CAD build for the part. Positions are in the model's coordinates, mm. A direction names the side the tool comes from. Round coordinates to 2 decimals unless told otherwise and drop trailing zeros. Loops run counter-clockwise (first coordinate to the right, second up) from the corner with the lowest first, then second, coordinate; pieces in that order, holes last.
Autodesk Inventor part; units mm, degrees
ref_plane "YZ Plane" through (0, 0, 0) normal (1, 0, 0) x (0, 1, 0)
ref_plane "XZ Plane" through (0, 0, 0) normal (0, 1, 0) x (-1, 0, 0)
ref_plane "XY Plane" through (0, 0, 0) normal (0, 0, 1) x (1, 0, 0)
sketch "main box1" plane through (0, 0, 0) normal (0, 1, 0) x (-1, 0, 0)
  line L0 (11.2873, -1.2021) -> (241.2873, -1.2021)
  line L1 (241.2873, -1.2021) -> (241.2873, -171.2021)
  line L2 (241.2873, -171.2021) -> (11.2873, -171.2021)
  line L3 (11.2873, -171.2021) -> (11.2873, -1.2021)
  point P0 (0, 0)
  dimension "d2" = 230
  dimension "d3" = 170
extrude "Main box" add sketch "main box1" along normal blind 50
sketch "Ethernet1" plane through (-11.2873, 0, -1.2021) normal (1, 0, 0) x (0, 0, -1)
  line L0 (16, 27.2) -> (30, 27.2)
  line L1 (31, 26.2) -> (31, 13)
  line L2 (30, 12) -> (16, 12)
  line L3 (15, 13) -> (15, 26.2)
  line L4 (0, 0) -> (170, 0)
  line L5 (0, 0) -> (0, 50)
  arc A0 (16, 27.2) -> (15, 26.2) centre (16, 26.2) ccw
  arc A1 (15, 13) -> (16, 12) centre (16, 13) ccw
  arc A2 (30, 12) -> (31, 13) centre (30, 13) ccw
  arc A3 (31, 26.2) -> (30, 27.2) centre (30, 26.2) ccw
  line L6 (46, 27.2) -> (60, 27.2)
  line L7 (61, 26.2) -> (61, 13)
  line L8 (60, 12) -> (46, 12)
  line L9 (45, 13) -> (45, 26.2)
  arc A4 (46, 27.2) -> (45, 26.2) centre (46, 26.2) ccw
  arc A5 (45, 13) -> (46, 12) centre (46, 13) ccw
  arc A6 (60, 12) -> (61, 13) centre (60, 13) ccw
  arc A7 (61, 26.2) -> (60, 27.2) centre (60, 26.2) ccw
  arc A8 (76, 27.2) -> (75, 26.2) centre (76, 26.2) ccw
  arc A9 (75, 13) -> (76, 12) centre (76, 13) ccw
  line L10 (76, 27.2) -> (90, 27.2)
  arc A10 (91, 26.2) -> (90, 27.2) centre (90, 26.2) ccw
  line L11 (91, 26.2) -> (91, 13)
  line L12 (90, 12) -> (76, 12)
  arc A11 (90, 12) -> (91, 13) centre (90, 13) ccw
  line L13 (75, 13) -> (75, 26.2)
  arc A12 (106, 27.2) -> (105, 26.2) centre (106, 26.2) ccw
  line L14 (105, 13) -> (105, 26.2)
  arc A13 (105, 13) -> (106, 12) centre (106, 13) ccw
  line L15 (106, 27.2) -> (120, 27.2)
  line L16 (120, 12) -> (106, 12)
  arc A14 (121, 26.2) -> (120, 27.2) centre (120, 26.2) ccw
  line L17 (121, 26.2) -> (121, 13)
  arc A15 (120, 12) -> (121, 13) centre (120, 13) ccw
  point P0 (-1.2021, 0)
  point P1 (15, 27.2)
  point P2 (31, 12)
  point P3 (31, 27.2)
  point P4 (15, 12)
  point P5 (45, 27.2)
  point P6 (61, 12)
  point P7 (61, 27.2)
  point P8 (45, 12)
  point P9 (0, 25)
  point P10 (75, 27.2)
  point P11 (91, 27.2)
  point P12 (91, 12)
  point P13 (75, 12)
  point P14 (105, 27.2)
  point P15 (105, 12)
  point P16 (121, 27.2)
  point P17 (121, 12)
  dimension "d6" = 16
  dimension "d7" = 15.2
  dimension "d98" = 12
  dimension "d99" = 15
  dimension "d100" = 1
  dimension "d103" = 1
  dimension "d104" = 45
  dimension "d107" = 1
  dimension "d110" = 1
  dimension "d111" = 75
  dimension "d112" = 105
extrude "Ethernet" cut sketch "Ethernet1" against normal blind 20
sketch "wheel 4 port connection" plane through (0, 50, 0) normal (0, 1, 0) x (1, 0, 0)
  line L0 (-216.7873, 22.7021) -> (-227.7873, 22.7021)
  line L1 (-228.7873, 21.7021) -> (-228.7873, 14.7021)
  line L2 (-227.7873, 13.7021) -> (-216.7873, 13.7021)
  line L3 (-215.7873, 14.7021) -> (-215.7873, 21.7021)
  line L4 (-241.2873, 171.2021) -> (-241.2873, 1.2021)
  line L5 (-241.2873, 1.2021) -> (-11.2873, 1.2021)
  arc A0 (-227.7873, 22.7021) -> (-228.7873, 21.7021) centre (-227.7873, 21.7021) ccw
  arc A1 (-215.7873, 21.7021) -> (-216.7873, 22.7021) centre (-216.7873, 21.7021) ccw
  arc A2 (-216.7873, 13.7021) -> (-215.7873, 14.7021) centre (-216.7873, 14.7021) ccw
  arc A3 (-228.7873, 14.7021) -> (-227.7873, 13.7021) centre (-227.7873, 14.7021) ccw
  point P0 (0, 0)
  point P1 (-215.7873, 22.7021)
  point P2 (-228.7873, 13.7021)
  point P3 (-228.7873, 22.7021)
  point P4 (-215.7873, 13.7021)
  dimension "d22" = 13
  dimension "d23" = 9
  dimension "d76" = 12.5
  dimension "d77" = 12.5
  dimension "d113" = 1
extrude "wheel" cut sketch "wheel 4 port connection" against normal blind 20
sketch "Motor left 4 port connection" plane through (0, 50, 0) normal (0, 1, 0) x (1, 0, 0)
  line L0 (-181.7873, 22.7021) -> (-192.7873, 22.7021)
  line L1 (-193.7873, 21.7021) -> (-193.7873, 14.7021)
  line L2 (-192.7873, 13.7021) -> (-181.7873, 13.7021)
  line L3 (-180.7873, 14.7021) -> (-180.7873, 21.7021)
  line L4 (-241.2873, 1.2021) -> (-11.2873, 1.2021)
  line L5 (-215.7873, 21.7021) -> (-215.7873, 14.7021)
  arc A0 (-180.7873, 21.7021) -> (-181.7873, 22.7021) centre (-181.7873, 21.7021) ccw
  arc A1 (-181.7873, 13.7021) -> (-180.7873, 14.7021) centre (-181.7873, 14.7021) ccw
  arc A2 (-193.7873, 14.7021) -> (-192.7873, 13.7021) centre (-192.7873, 14.7021) ccw
  arc A3 (-192.7873, 22.7021) -> (-193.7873, 21.7021) centre (-192.7873, 21.7021) ccw
  point P0 (0, 0)
  point P1 (-180.7873, 22.7021)
  point P2 (-193.7873, 13.7021)
  point P3 (-193.7873, 22.7021)
  point P4 (-180.7873, 13.7021)
  point P5 (-221.7873, 20.7021)
  point P6 (-221.7873, 13.7021)
  point P7 (-215.7873, 14.7021)
  dimension "d26" = 13
  dimension "d27" = 9
  dimension "d78" = 12.5
  dimension "d79" = 22
  dimension "d114" = 1
extrude "Motor left" cut sketch "Motor left 4 port connection" against normal blind 20
sketch "Motor right 4 port connection" plane through (0, 50, 0) normal (0, 1, 0) x (1, 0, 0)
  line L0 (-192.7873, 44.7021) -> (-181.7873, 44.7021)
  line L1 (-180.7873, 45.7021) -> (-180.7873, 52.7021)
  line L2 (-181.7873, 53.7021) -> (-192.7873, 53.7021)
  line L3 (-193.7873, 52.7021) -> (-193.7873, 45.7021)
  line L4 (-192.7873, 22.7021) -> (-181.7873, 22.7021)
  line L5 (-193.7873, 14.7021) -> (-193.7873, 21.7021)
  arc A0 (-192.7873, 53.7021) -> (-193.7873, 52.7021) centre (-192.7873, 52.7021) ccw
  arc A1 (-180.7873, 52.7021) -> (-181.7873, 53.7021) centre (-181.7873, 52.7021) ccw
  arc A2 (-181.7873, 44.7021) -> (-180.7873, 45.7021) centre (-181.7873, 45.7021) ccw
  arc A3 (-193.7873, 45.7021) -> (-192.7873, 44.7021) centre (-192.7873, 45.7021) ccw
  point P0 (0, 0)
  point P1 (-193.7873, 44.7021)
  point P2 (-180.7873, 53.7021)
  point P3 (-180.7873, 44.7021)
  point P4 (-193.7873, 53.7021)
  point P5 (-198.7873, 20.7021)
  point P6 (-191.7873, 20.7021)
  point P7 (-198.7873, 13.7021)
  point P8 (-181.7873, 22.7021)
  dimension "d30" = 13
  dimension "d31" = 9
  dimension "d80" = 22
  dimension "d115" = 1
extrude "Motor right" cut sketch "Motor right 4 port connection" against normal blind 20
sketch "Sketch10" plane through (0, 50, 0) normal (0, 1, 0) x (1, 0, 0)
  circle A0 centre (-157.2873, 18.2021) radius 4
  line L0 (-241.2873, 1.2021) -> (-11.2873, 1.2021)
  circle A1 centre (-157.2873, 48.2021) radius 4
  circle A2 centre (-157.2873, 78.2021) radius 4
  line L1 (-157.2873, 18.2021) -> (-157.2873, 78.2021) construction
  line L2 (-181.7873, 13.7021) -> (-192.7873, 13.7021) construction
  line L3 (-180.7873, 21.7021) -> (-180.7873, 14.7021) construction
  line L4 (-180.7873, 18.2021) -> (-157.2873, 18.2021) construction
  arc A3 (-193.7873, 14.7021) -> (-192.7873, 13.7021) centre (-192.7873, 14.7021) ccw construction
  arc A4 (-192.7873, 22.7021) -> (-193.7873, 21.7021) centre (-192.7873, 21.7021) ccw construction
  line L5 (-193.7873, 14.7021) -> (-193.7873, 21.7021) construction
  arc A5 (-193.7873, 14.7021) -> (-192.7873, 13.7021) centre (-192.7873, 14.7021) ccw construction
  line L6 (-181.7873, 13.7021) -> (-192.7873, 13.7021) construction
  arc A6 (-181.7873, 13.7021) -> (-180.7873, 14.7021) centre (-181.7873, 14.7021) ccw construction
  line L7 (-180.7873, 21.7021) -> (-180.7873, 14.7021) construction
  arc A7 (-180.7873, 21.7021) -> (-181.7873, 22.7021) centre (-181.7873, 21.7021) ccw construction
  line L8 (-192.7873, 22.7021) -> (-181.7873, 22.7021) construction
  point P0 (0, 0)
  point P1 (-187.2873, 13.7021)
  point P2 (-187.2873, 13.7021)
  dimension "d34" = 8
  dimension "d86" = 30
  dimension "d87" = 30
  dimension "d88" = 30
extrude "PD" cut sketch "Sketch10" against normal blind 20
sketch "Power socket" plane through (0, 50, 0) normal (0, 1, 0) x (1, 0, 0)
  circle A0 centre (-221.2873, 107.2021) radius 6.5
  line L0 (-241.2873, 171.2021) -> (-241.2873, 1.2021)
  circle A1 centre (-221.2873, 129.2021) radius 6.5
  circle A2 centre (-221.2873, 151.2021) radius 6.5
  circle A3 centre (-199.2873, 151.2021) radius 6.5
  circle A4 centre (-199.2873, 129.2021) radius 6.5
  circle A5 centre (-199.2873, 107.2021) radius 6.5
  circle A6 centre (-177.2873, 151.2021) radius 6.5
  circle A7 centre (-177.2873, 129.2021) radius 6.5
  circle A8 centre (-177.2873, 107.2021) radius 6.5
  line L1 (-11.2873, 171.2021) -> (-241.2873, 171.2021)
  line L2 (-221.2873, 107.2021) -> (-221.2873, 151.2021) construction
  line L3 (-221.2873, 151.2021) -> (-177.2873, 151.2021) construction
  line L4 (-177.2873, 151.2021) -> (-177.2873, 107.2021) construction
  line L5 (-177.2873, 107.2021) -> (-221.2873, 107.2021) construction
  line L6 (-221.2873, 129.2021) -> (-177.2873, 129.2021) construction
  line L7 (-199.2873, 151.2021) -> (-199.2873, 107.2021) construction
  point P0 (0, 0)
  dimension "d43" = 13
  dimension "d90" = 20
  dimension "d94" = 20
  dimension "d95" = 22
  dimension "d96" = 22
extrude "Power" cut sketch "Power socket" against normal blind 20
sketch "Sketch22" plane through (0, 0, 0) normal (0, -1, 0) x (1, 0, 0)
  line L0 (-19.2873, -9.2021) -> (-233.2873, -9.2021)
  line L1 (-233.2873, -9.2021) -> (-233.2873, -163.2021)
  line L2 (-233.2873, -163.2021) -> (-19.2873, -163.2021)
  line L3 (-19.2873, -163.2021) -> (-19.2873, -9.2021)
  line L4 (-241.2873, -1.2021) -> (-11.2873, -1.2021)
  line L5 (-11.2873, -171.2021) -> (-241.2873, -171.2021)
  line L6 (-11.2873, -1.2021) -> (-11.2873, -171.2021)
  line L7 (-241.2873, -171.2021) -> (-241.2873, -1.2021)
  point P0 (0, 0)
  dimension "d70" = 8
  dimension "d71" = 8
  dimension "d72" = 8
  dimension "d73" = 8
extrude "Extrusion21" cut sketch "Sketch22" against normal blind 42 contours L3 L2 L1 L0
sketch "Sketch23" plane through (-11.2873, 0, -1.2021) normal (1, 0, 0) x (0, 0, -1)
  circle A0 centre (145, 25) radius 12.5
  line L0 (0, 0) -> (170, 0)
  line L1 (170, 0) -> (170, 50)
  point P0 (-1.2021, 0)
  dimension "d117" = 25
  dimension "d118" = 25
  dimension "d119" = 25
extrude "Extrusion22" cut sketch "Sketch23" against normal blind 20
properties part number "BreakoutBox"
Item 1: 3-axis set-ups, long thin cutter, end or side, ignore diameter. For faces 5 (the flat face through (-187, 46, -13.702)), 6 (the flat face through (-125, 50, -85)), 7 (the flat face through (-15, 12, -114)): which of +Z, -Z, +X, -X, +Y, -Y reach the whole face in a straight line?
Verdict:
face 5: +Y, -Y
face 6: +Z, -Z, +X, -X, +Y
face 7: +X
Item 2: Mould opens along X. For faces 1 (the flat face through (-125, 25, -1.202)), 2 (the flat face through (-241.287, 25, -85)), 3 (the flat face through (-11.287, 30, -87)), 4 (the flat face through (-128, 21, -163.202)) say: released by +X, released by -X, zero draft, split by the parting line, or undercut.
Verdict:
face 1: zero draft
face 2: released by -X
face 3: released by +X
face 4: undercut
Item 3: Cut at B-B (x = -59.5). List the corners of the cut face in (y, z), plus the area to 3 significant figures.
Verdict:
outline: (0, -171.2) - (50, -171.2) - (50, -1.2) - (0, -1.2) - (0, -9.2) - (42, -9.2) - (42, -163.2) - (0, -163.2) - close
area: 2,030 mm2
Item 4: Cut at C-C (x = -225). List the corners of the cut face in (y, z).
Verdict:
outline: (0, -171.2) - (50, -171.2) - (50, -156.54) - (42, -156.54) - (42, -163.2) - (0, -163.2) - close; (0, -9.2) - (42, -9.2) - (42, -13.7) - (50, -13.7) - (50, -1.2) - (0, -1.2) - close; (42, -145.87) - (50, -145.87) - (50, -134.54) - (42, -134.54) - close; (42, -123.87) - (50, -123.87) - (50, -112.54) - (42, -112.54) - close; (42, -101.87) - (50, -101.87) - (50, -22.7) - (42, -22.7) - close
Item 5: Cut at D-D (z = -68). List the corners of the cut face in (x, y), plus the area to 3 significant figures.
Verdict:
outline: (-241.29, 0) - (-233.29, 0) - (-233.29, 42) - (-19.29, 42) - (-19.29, 0) - (-11.29, 0) - (-11.29, 50) - (-241.29, 50) - close
area: 2,510 mm2
Item 6: Flat gauge pins, fed straight in: P1, Ø1, axis at y = 14, z = -116.5, coming from the +X side; P2, Ø15, axis at x = -221.29, z = -129.2, coming from the -Y side. Where does each tip first touch, or does it go through?
Verdict:
P1: stops at x = -233.29
P2: stops at y = 42
Item 7: Wall check: L1, parallel to Z at x = -186, y = 39; L2, parallel to X at y = 21, z = -45; L3, parallel to Z at x = -154, y = 42.5. Give the ranges that are in metal, low to high.
Verdict:
L1: z = -171.2 to -163.2, -9.2 to -1.2
L2: x = -241.29 to -233.29, -19.29 to -11.29
L3: z = -171.2 to -80.48, -75.92 to -50.48, -45.92 to -20.48, -15.92 to -1.2
Item 8: Cut at A-A (z = -126). List the corners of the cut face in (x, y), plus the area to 3 significant figures.
Verdict:
outline: (-241.29, 0) - (-233.29, 0) - (-233.29, 42) - (-226.94, 42) - (-226.94, 50) - (-241.29, 50) - close; (-215.63, 42) - (-204.94, 42) - (-204.94, 50) - (-215.63, 50) - close; (-193.63, 42) - (-182.94, 42) - (-182.94, 50) - (-193.63, 50) - close; (-171.63, 42) - (-19.29, 42) - (-19.29, 0) - (-11.29, 0) - (-11.29, 50) - (-171.63, 50) - close
area: 2,240 mm2
